Print and shaded views of the part. All mm, measured from the part's lowest x, y and z. A direction names the side the tool comes from. Round coordinates to 2 decimals unless told otherwise and drop trailing zeros. Loops run counter-clockwise (first coordinate to the right, second up) from the corner with the lowest first, then second, coordinate; pieces in that order, holes last. Notation, with made-up numbers: (42.5, 19) - (97.5, 19) arc R16 cw to (97.5, 32) - close; hole circle Ø7 at (56, 7). An arc over 180 degrees is marked (long way). Answer as a JSON object with one key per item and string values.
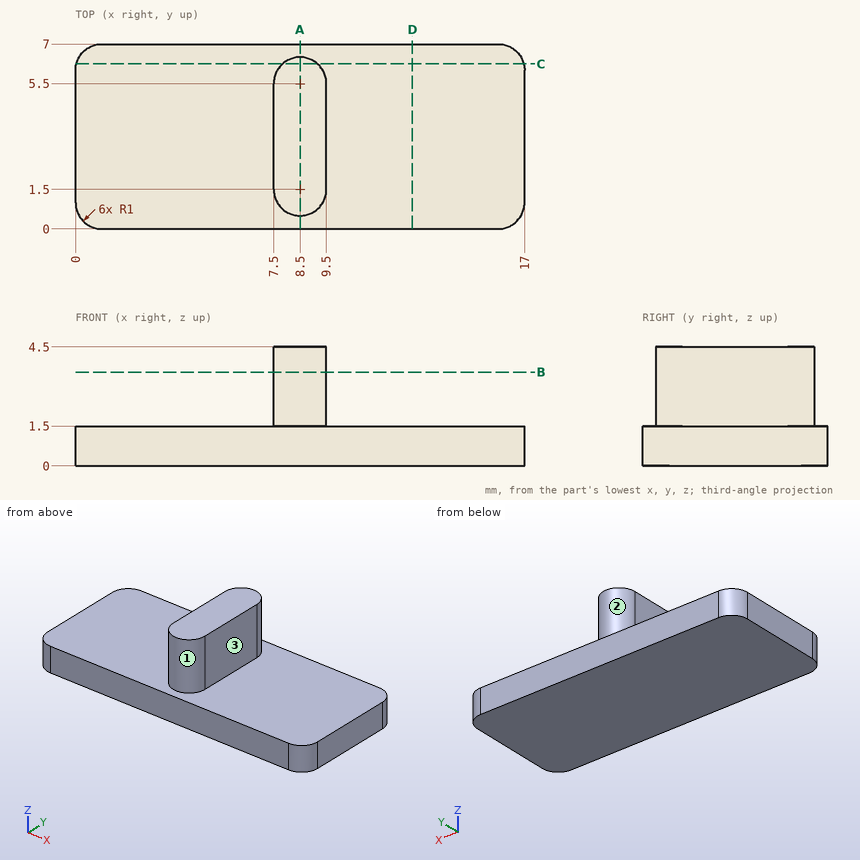
1) Slice it at B-B on z = 3.55. List the corners of the cut face in (x, y).
Values follow:
{"outline": "(7.5, 1.5) arc R1 ccw to (9.5, 1.5) - (9.5, 5.5) arc R1 ccw to (7.5, 5.5) - close"}
2) Slice it at A-A on x = 8.5. List the corners of the cut face in (y, z).
Values follow:
{"outline": "(0, 0) - (7, 0) - (7, 1.5) - (6.5, 1.5) - (6.5, 4.5) - (0.5, 4.5) - (0.5, 1.5) - (0, 1.5) - close"}
3) Probe probe 1 along X at (y, z) = (4.5, 3.85); probe 2 along Z at (x, y) = (6, 2.5); probe 3 along X at (y, z) = (0.75, 4.3). List the from-to ranges inside material, lowest first.
Values follow:
{"probe 1": "7.5 to 9.5", "probe 2": "0 to 1.5", "probe 3": "7.84 to 9.16"}
4) Slice it at C-C on y = 6.25. List the corners of the cut face in (x, z).
Values follow:
{"outline": "(0.03, 0) - (16.97, 0) - (16.97, 1.5) - (9.16, 1.5) - (9.16, 4.5) - (7.84, 4.5) - (7.84, 1.5) - (0.03, 1.5) - close"}
5) Tool access for the marked faces 1, 2 and 3: list every direction of +Z, -Z, +X, -X, +Y, -Y with a clear straight run to the whole face (end or side of a thin tool).
Values follow:
{"face 1": "+Z, -Y", "face 2": "+Z, +Y", "face 3": "+Z, +X, +Y, -Y"}
6) Slice it at D-D on x = 12.75. List the corners of the cut face in (y, z), then the cut area to 3 significant figures.
Values follow:
{"outline": "(0, 0) - (7, 0) - (7, 1.5) - (0, 1.5) - close", "area": "10.5 mm²"}
7) Drop flat-ended pins along their axis: P1, Ø0.9, axis at y = 4.5, z = 3, coming from the +X side; P2, Ø0.9, axis at y = 4, z = 3, coming from the -X side. Give the stop position or say it passes through.
Values follow:
{"P1": "x = 9.5", "P2": "x = 7.5"}
